Model file for the job. Use its own axes, mm. A direction names the side the tool comes from. Round coordinates to 2 decimals unless told otherwise and drop trailing zeros. Order: outer loops, then holes, each group sorted by start corner. A loop starts at its lowest first (then second) coordinate and runs counter-clockwise, first axis right, second up. Notation, with made-up numbers: (25, -39.75) -> (83, -39.75) arc R21 cw to (83, -19.75) -> close; hole circle Ø4 at (37, -30.5). An arc over 180 degrees is marked (long way). Put each result on its own line as item: value. Start each with the question number.
Q1. Cut at A-A, the plane y = 41.5. List the corners of the cut face in (x, z), and give its area (3 significant figures).
Q2. Cut at B-B, the plane z = -10. List the corners of the cut face in (x, y).
Q3. Pull direction X, two halves, no side cores. Call faces 1 (the face through (-4, 0, -33)), 2 (the face through (0, -2, -31)), 3 (the face through (-10, 36, -23)), 4 (the face through (-12, -16, -26)): released by +X, released by -X, zero draft, split by the parting line, or undercut.
Q4. Cut at C-C, the plane x = 0. State how many separate pieces and enclosed holes the cut face has, and give its area (3 significant figures).
Q5. 3-axis set-ups, long thin cutter, end or side, ignore diameter. For faces 5 (the face through (0, 50, -15)), 6 (the face through (10, 36, 3)), 7 (the face through (1.69, 2.66, -31.48)), 8 (the face through (-3.157, -14.216, -24.687)): which of +Z, -Z, +X, -X, +Y, -Y reach the whole face in a straight line?
Q6. Cut at D-D, the plane y = 0. List the corners of the cut face in (x, z).
Q7. Flat gauge pins, fed straight in: P1, Ø4, axis at x = -4.5, y = -9.5, coming from the +Z side; P2, Ø16, axis at x = -4, z = -10, coming from the -Y side; P3, Ø11.5, axis at y = 32, z = -12.5, coming from the -X side; P4, Ø19, axis at y = 28, z = -4, coming from the +X side. Where does each tip first touch, or does it go through?
Q8. Probe L1, parallel to Y at x = 0, z = 4.5; L2, parallel to X at y = 0, z = -31; L3, parallel to Z at x = 8, y = 45. List the from-to ranges inside material, lowest first.
Autodesk Inventor part; units mm, degrees
ref_plane "YZ Plane" through (0, 0, 0) normal (1, 0, 0) x (0, 1, 0)
ref_plane "XZ Plane" through (0, 0, 0) normal (0, 1, 0) x (-1, 0, 0)
ref_plane "XY Plane" through (0, 0, 0) normal (0, 0, 1) x (1, 0, 0)
sketch "Sketch1" plane through (0, 0, 0) normal (0, 0, 1) x (1, 0, 0)
  circle A0 centre (0, 0) radius 14.25
  circle A1 centre (0, 0) radius 20
  line L0 (0, 50) -> (10, 50)
  line L1 (10, 50) -> (10, 17.3205)
  line L2 (0, 20) -> (0, 50)
  line L3 (0, 50) -> (-10, 50)
  line L4 (-10, 50) -> (-10, 17.3205)
  point P0 (-20, 0)
  point P1 (20, 0)
  dimension "d0" = 28.5
  dimension "d1" = 40
  dimension "d25" = 10
  dimension "d31" = 10
extrude "Extrusion1" add sketch "Sketch1" along normal blind 10
ref_plane "Work Plane1" through (0, 0, -10) normal (0, 0, 1) x (1, 0, 0)
mirror "Mirror1" about plane through (0, 0, -10) normal (0, 0, 1) of "Extrusion1"
sketch "Sketch2" plane through (0, 0, -30) normal (0, 0, -1) x (-1, 0, 0)
  circle A0 centre (0, 0) radius 14.25
  circle A1 centre (0, 0) radius 20
  dimension "d11" = 40
extrude "Extrusion2" add sketch "Sketch2" along normal blind 3 contours A0 | A1
sketch "Sketch3" plane through (0, 0, -30) normal (0, 0, 1) x (1, 0, 0)
  circle A0 centre (0, 0) radius 3.15
  dimension "d14" = 6.3
extrude "Extrusion3" cut sketch "Sketch3" against normal blind 1
sketch "Sketch4" plane through (0, 0, -31) normal (0, 0, 1) x (1, 0, 0)
  circle A0 centre (0, 0) radius 3.15
  line L0 (0, 0) -> (0, -1.6)
  line L1 (0, -1.6) -> (-2.7134, -1.6)
  line L2 (0, -1.6) -> (2.7134, -1.6)
  dimension "d17" = 6.3
  dimension "d18" = 1.6
extrude "Extrusion4" cut sketch "Sketch4" against normal through all contours A0 L2 L1 picked at (-0.0447, 1.5505)
sketch "Sketch6" plane through (-7.5, 50, -22) normal (0, 1, 0) x (1, 0, 0)
  line L0 (17.5, 8) -> (17.5, 8)
  line L1 (17.5, -22) -> (17.5, -32)
  line L2 (-2.5, 8) -> (17.5, 8)
  line L3 (17.5, 8) -> (17.5, -32)
  line L4 (17.5, -32) -> (-2.5, -32)
  line L5 (-2.5, -32) -> (-2.5, 8)
  point P0 (7.5, -22)
extrude "Extrusion6" add sketch "Sketch6" along normal blind 5
sketch "Sketch7" plane through (-7.5, 55, -22) normal (0, 1, 0) x (1, 0, 0)
  line L0 (21.75, -32) -> (-6.75, -32)
  line L1 (7.5, -32) -> (7.5, 8)
  line L2 (10.65, 8) -> (4.35, 8)
  circle A0 centre (7.5, -12) radius 4.25
  point P0 (7.5, -22)
  dimension "d28" = 8.5
extrude "Extrusion7" cut sketch "Sketch7" against normal up to next
chamfer "Chamfer1" distance 5 angle 45 1 edges at (-14.25, 0, -20)
equation "\"d4\" = d25"
equation "\"BendRadius\" = Thickness"
equation "\"BendReliefWidth\" = Thickness"
equation "\"BendReliefDepth\" = 0.5 * Thickness"
equation "\"CornerReliefSize\" = 4 * Thickness"
equation "\"MinimumRemnant\" = 2 * Thickness"
equation "\"TransitionRadius\" = BendRadius"
equation "\"JacobiRadiusSize\" = BendRadius"
equation "\"GapSize\" = Thickness"
properties part number "baseRotor1"
Ans:
1. outline: (-10, -30) -> (10, -30) -> (10, -20) -> (-10, -20) -> close; (-10, 0) -> (10, 0) -> (10, 10) -> (-10, 10) -> close
1. area: 400 mm^2
2. outline: (-10, 50) -> (-4.25, 50) -> (-4.25, 55) -> (-10, 55) -> close; (4.25, 50) -> (10, 50) -> (10, 55) -> (4.25, 55) -> close
3. face 1: zero draft
3. face 2: undercut
3. face 3: released by -X
3. face 4: split by the parting line
4. separate pieces: 4
4. enclosed holes: 0
4. area: 1,070 mm^2
5. face 5: +X, -X, -Y
5. face 6: +Z, -Z, +X, +Y
5. face 7: +Z
5. face 8: none
6. outline: (-20, -33) -> (-3.15, -33) -> (-3.15, -30) -> (-14.25, -30) -> (-14.25, -25) -> (-19.25, -20) -> (-20, -20) -> close; (-20, 0) -> (-14.25, 0) -> (-14.25, 10) -> (-20, 10) -> close; (3.15, -33) -> (20, -33) -> (20, -20) -> (19.25, -20) -> (14.25, -25) -> (14.25, -30) -> (3.15, -30) -> close; (14.25, 0) -> (20, 0) -> (20, 10) -> (14.25, 10) -> close
7. P1: stops at z = -30
7. P2: stops at y = 50
7. P3: passes through
7. P4: stops at x = 10
8. L1: y = -20 to -14.25, 14.25 to 55
8. L2: x = -20 to -3.15, 3.15 to 20
8. L3: z = -30 to -20, 0 to 10
